```python
from build123d import *

# Parameters (mm, degrees)
F0_W     = 38.1
F0_H     = 25.3
F1_DEPTH = 3
F0_W_2   = 44.1
F0_H_2   = 31.3
F2_DEPTH = 6
F3_DEPTH = 6
F4_SIZE  = 0.6
F5_R     = 2


# Not quite as in the source:
# - a feature names something its author has since deleted; it is built from what else it names


with BuildPart() as f1:
    # F0 (on Front) → F1 (new body)
    with BuildSketch(Plane.XZ):
        Rectangle(F0_W, F0_H)
        with BuildLine():
            ThreePointArc((-8.6746757864, 9), (0, 12.5), (8.6746757864, 9))
            Line((8.6746757864, 9), (12.5, 9))
            Line((12.5, 9), (12.5, 0))
            Line((12.5, 0), (12.5, -9))
            Line((12.5, -9), (8.6746757864, -9))
            ThreePointArc((8.6746757864, -9), (0, -12.5), (-8.6746757864, -9))
            Line((-8.6746757864, -9), (-12.5, -9))
            Line((-12.5, -9), (-12.5, 0))
            Line((-12.5, 0), (-12.5, 9))
            Line((-12.5, 9), (-8.6746757864, 9))
        make_face(mode=Mode.SUBTRACT)
        with BuildLine():
            ThreePointArc((-3.0413812651, 9), (0, 9.5), (3.0413812651, 9))
            Line((3.0413812651, 9), (8.6746757864, 9))
            ThreePointArc((8.6746757864, 9), (0, 12.5), (-8.6746757864, 9))
            Line((-8.6746757864, 9), (-3.0413812651, 9))
        make_face()
        with BuildLine():
            ThreePointArc((12.5, 0), (11.5039872942, -4.8896090165), (8.6746757864, -9))
            Line((8.6746757864, -9), (12.5, -9))
            Line((12.5, -9), (12.5, 0))
        make_face()
        with BuildLine():
            Line((8.6746757864, -9), (3.0413812651, -9))
            ThreePointArc((3.0413812651, -9), (0, -9.5), (-3.0413812651, -9))
            Line((-3.0413812651, -9), (-8.6746757864, -9))
            ThreePointArc((-8.6746757864, -9), (0, -12.5), (8.6746757864, -9))
        make_face()
        with BuildLine():
            Line((-12.5, -9), (-8.6746757864, -9))
            ThreePointArc((-8.6746757864, -9), (-11.5039872942, -4.8896090165), (-12.5, 0))
            Line((-12.5, 0), (-12.5, -9))
        make_face()
        with BuildLine():
            Line((-3.0413812651, 9), (3.0413812651, 9))
            ThreePointArc((3.0413812651, 9), (0, 9.5), (-3.0413812651, 9))
        make_face()
        with BuildLine():
            ThreePointArc((-3.0413812651, -9), (0, -9.5), (3.0413812651, -9))
            Line((3.0413812651, -9), (-3.0413812651, -9))
        make_face()
        with BuildLine():
            ThreePointArc((-6.4036735124, 7.0173332219), (-4.8254540539, 8.1832141102), (-3.0413812651, 9))
            Line((-3.0413812651, 9), (-8.6746757864, 9))
            ThreePointArc((-8.6746757864, 9), (-11.5039872942, 4.8896090165), (-12.5, 0))
            ThreePointArc((-12.5, 0), (-11.5039872942, -4.8896090165), (-8.6746757864, -9))
            Line((-8.6746757864, -9), (-3.0413812651, -9))
            ThreePointArc((-3.0413812651, -9), (-4.8254540539, -8.1832141102), (-6.4036735124, -7.0173332219))
            ThreePointArc((-6.4036735124, -7.0173332219), (-7.9193096463, -7.2857878881), (-8.7654599313, -6))
            Line((-8.7654599313, -6), (-9.5, -6))
            Line((-9.5, -6), (-9.5, 0))
            Line((-9.5, 0), (-9.5, 6))
            Line((-9.5, 6), (-8.7654599313, 6))
            ThreePointArc((-8.7654599313, 6), (-7.9193096463, 7.2857878881), (-6.4036735124, 7.0173332219))
        make_face()
        with BuildLine():
            Line((9.5, 6), (9.5, 0))
            Line((9.5, 0), (9.5, -6))
            Line((9.5, -6), (8.7654599313, -6))
            ThreePointArc((8.7654599313, -6), (7.9193096463, -7.2857878881), (6.4036735124, -7.0173332219))
            ThreePointArc((6.4036735124, -7.0173332219), (4.8254540539, -8.1832141102), (3.0413812651, -9))
            Line((3.0413812651, -9), (8.6746757864, -9))
            ThreePointArc((8.6746757864, -9), (11.5039872942, -4.8896090165), (12.5, 0))
            ThreePointArc((12.5, 0), (11.5039872942, 4.8896090165), (8.6746757864, 9))
            Line((8.6746757864, 9), (3.0413812651, 9))
            ThreePointArc((3.0413812651, 9), (4.8254540539, 8.1832141102), (6.4036735124, 7.0173332219))
            ThreePointArc((6.4036735124, 7.0173332219), (7.9193096463, 7.2857878881), (8.7654599313, 6))
            Line((8.7654599313, 6), (9.5, 6))
        make_face()
        with BuildLine():
            Line((9.5, -6), (9.5, 0))
            ThreePointArc((9.5, 0), (9.1607649693, -2.5160256709), (8.1672873313, -4.852362069))
            ThreePointArc((8.1672873313, -4.852362069), (8.6069425852, -5.3529135915), (8.7654599313, -6))
            Line((8.7654599313, -6), (9.5, -6))
        make_face()
        with BuildLine():
            ThreePointArc((-8.7654599313, -6), (-8.6069425852, -5.3529135915), (-8.1672873313, -4.852362069))
            ThreePointArc((-8.1672873313, -4.852362069), (-9.1607649693, -2.5160256709), (-9.5, 0))
            Line((-9.5, 0), (-9.5, -6))
            Line((-9.5, -6), (-8.7654599313, -6))
        make_face()
        with BuildLine():
            ThreePointArc((-9.5, 0), (-9.1607649693, 2.5160256709), (-8.1672873313, 4.852362069))
            ThreePointArc((-8.1672873313, 4.852362069), (-8.6069425852, 5.3529135915), (-8.7654599313, 6))
            Line((-8.7654599313, 6), (-9.5, 6))
            Line((-9.5, 6), (-9.5, 0))
        make_face()
        with BuildLine():
            ThreePointArc((8.1672873313, 4.852362069), (9.1607649693, 2.5160256709), (9.5, 0))
            Line((9.5, 0), (9.5, 6))
            Line((9.5, 6), (8.7654599313, 6))
            ThreePointArc((8.7654599313, 6), (8.6069425852, 5.3529135915), (8.1672873313, 4.852362069))
        make_face()
        with BuildLine():
            ThreePointArc((-12.5, 0), (-11.5039872942, 4.8896090165), (-8.6746757864, 9))
            Line((-8.6746757864, 9), (-12.5, 9))
            Line((-12.5, 9), (-12.5, 0))
        make_face()
        with BuildLine():
            Line((12.5, 9), (8.6746757864, 9))
            ThreePointArc((8.6746757864, 9), (11.5039872942, 4.8896090165), (12.5, 0))
            Line((12.5, 0), (12.5, 9))
        make_face()
        with BuildLine():
            ThreePointArc((5.9654599313, 6), (6.0796720432, 6.5538497149), (6.4036735124, 7.0173332219))
            ThreePointArc((6.4036735124, 7.0173332219), (4.8254540539, 8.1832141102), (3.0413812651, 9))
            Line((3.0413812651, 9), (-3.0413812651, 9))
            ThreePointArc((-3.0413812651, 9), (-4.8254540539, 8.1832141102), (-6.4036735124, 7.0173332219))
            ThreePointArc((-6.4036735124, 7.0173332219), (-6.0796720432, 6.5538497149), (-5.9654599313, 6))
            Line((-5.9654599313, 6), (5.9654599313, 6))
        make_face()
        with BuildLine():
            ThreePointArc((3.0413812651, -9), (4.8254540539, -8.1832141102), (6.4036735124, -7.0173332219))
            ThreePointArc((6.4036735124, -7.0173332219), (6.0796720432, -6.5538497149), (5.9654599313, -6))
            Line((5.9654599313, -6), (-5.9654599313, -6))
            ThreePointArc((-5.9654599313, -6), (-6.0796720432, -6.5538497149), (-6.4036735124, -7.0173332219))
            ThreePointArc((-6.4036735124, -7.0173332219), (-4.8254540539, -8.1832141102), (-3.0413812651, -9))
            Line((-3.0413812651, -9), (3.0413812651, -9))
        make_face()
    extrude(amount=F1_DEPTH)

    # F0 (on Front) → F2 (join)
    with BuildSketch(Plane.XZ):
        Rectangle(F0_W_2, F0_H_2)
        Rectangle(F0_W, F0_H, mode=Mode.SUBTRACT)
    extrude(amount=F2_DEPTH)

    # F0 (on Front) → F3 (join)
    with BuildSketch(Plane.XZ):
        Rectangle(F0_W_2, F0_H_2)
        Rectangle(F0_W, F0_H, mode=Mode.SUBTRACT)
    extrude(amount=-F3_DEPTH)

    # F4
    f4_edges = [f1.edges().sort_by_distance(p)[0] for p in [
        (-19.05, -6, 0),
        (0, -6, -12.65),
        (0, -6, 12.65),
        (19.05, -6, 0),
    ]]
    chamfer(f4_edges, length=F4_SIZE)

    # F5
    f5_edges = [f1.edges().sort_by_distance(p)[0] for p in [
        (22.05, 0, 15.65),
        (22.05, 0, -15.65),
        (-22.05, 0, -15.65),
        (-22.05, 0, 15.65),
    ]]
    fillet(f5_edges, radius=F5_R)


solid = f1.part
```
Verification items for the finished model (mm, model axes). A direction names the side the tool comes from. Coordinates: 2 decimals unless noted, no trailing zeros. Loops run counter-clockwise (first coordinate to the right, second up) from the corner with the lowest first, then second, coordinate; pieces in that order, holes last. Notation, with made-up numbers: (-36.75, -22.5) - (-20.75, -22.5) arc R16 ccw to (-20.75, -0.5) - close; hole circle Ø6 at (-34, -22). An arc over 180 degrees is marked (long way). Put each result on its own line as item: value.
Item 1: Scan lines: line 1 along Z through (x, y) = (16, -4.5); line 2 along X through (y, z) = (2.75, -10.5); line 3 along Z through (x, y) = (3, -2.25). Record each from-to range of solid material in increasing order.
Conclusion:
line 1: z = -15.65 to -12.65, 12.65 to 15.65
line 2: x = -22.05 to -19.05, 19.05 to 22.05
line 3: z = -15.65 to -6, 6 to 15.65
Item 2: Set-up check for faces 1 (the face through (0, 0, 15.65)), 2 (the face through (0, 0, -8)), 3 (the face through (-19.05, -4, 0)), 4 (the face through (0, -1, 6)), 5 (the face through (-21.48, 0.08, 15.05)): record each of +Z, -Z, +X, -X, +Y, -Y from which the full face is reachable in a straight line by a thin tool's end or side.
Conclusion:
face 1: +Z, +X, -X, +Y, -Y
face 2: +Y
face 3: -Y
face 4: +Y, -Y
face 5: +Z, -X, +Y, -Y
Item 3: Section check B-B (y = 4.75). Enter the section's corners in (x, z).
Conclusion:
outline: (-22.05, -13.65) arc R2 ccw to (-20.05, -15.65) - (20.05, -15.65) arc R2 ccw to (22.05, -13.65) - (22.05, 13.65) arc R2 ccw to (20.05, 15.65) - (-20.05, 15.65) arc R2 ccw to (-22.05, 13.65) - close; hole (-19.05, -12.65) - (19.05, -12.65) - (19.05, 12.65) - (-19.05, 12.65) - close
Item 4: Section check D-D (z = -4). Enter the section's corners in (x, y).
Conclusion:
outline: (-22.05, -6) - (-19.65, -6) - (-19.05, -5.4) - (-19.05, -3) - (-8.62, -3) - (-8.62, 0) - (-19.05, 0) - (-19.05, 6) - (-22.05, 6) - close; (8.62, -3) - (19.05, -3) - (19.05, -5.4) - (19.65, -6) - (22.05, -6) - (22.05, 6) - (19.05, 6) - (19.05, 0) - (8.62, 0) - close
Item 5: Section check A-A (x = -2.5). Enter the section's corners in (y, z).
Conclusion:
outline: (-6, -15.65) - (6, -15.65) - (6, -12.65) - (0, -12.65) - (0, -6) - (-3, -6) - (-3, -12.65) - (-5.4, -12.65) - (-6, -13.25) - close; (-6, 13.25) - (-5.4, 12.65) - (-3, 12.65) - (-3, 6) - (0, 6) - (0, 12.65) - (6, 12.65) - (6, 15.65) - (-6, 15.65) - close
Item 6: Gauge pin test, flat ends, axial feed: pin 1 Ø7.5 at (x, z) = (-2.5, 0) entering from +Y; pin 2 Ø3 at (x, z) = (-9.5, -8.5) entering from -Y; pin 3 Ø2 at (x, z) = (-3, -12) entering from -Y; pin 4 Ø2 at (x, z) = (-10.5, 9.5) entering from +Y. Record the tip position at first contact, or that the pin passes through.
Conclusion:
pin 1: passes through
pin 2: stops at y = -3
pin 3: stops at y = -5.75
pin 4: stops at y = 0
Item 7: Draft check along Z on faces 6 (the face through (-5, -6, -14)), 7 (the face through (0, 3, 12.65)), 8 (the face through (21.45, 0.08, 15.08)). Enter one of: pulls with the +Z half, pulls with the -Z half, needs draft (parallel to the pull), parting line crosses it, or undercut.
Conclusion:
face 6: needs draft
face 7: undercut
face 8: pulls with the +Z half
Item 8: Section check C-C (z = -8). Enter the section's corners in (x, y).
Conclusion:
outline: (-22.05, -6) - (-19.65, -6) - (-19.05, -5.4) - (-19.05, -3) - (19.05, -3) - (19.05, -5.4) - (19.65, -6) - (22.05, -6) - (22.05, 6) - (19.05, 6) - (19.05, 0) - (-19.05, 0) - (-19.05, 6) - (-22.05, 6) - close
